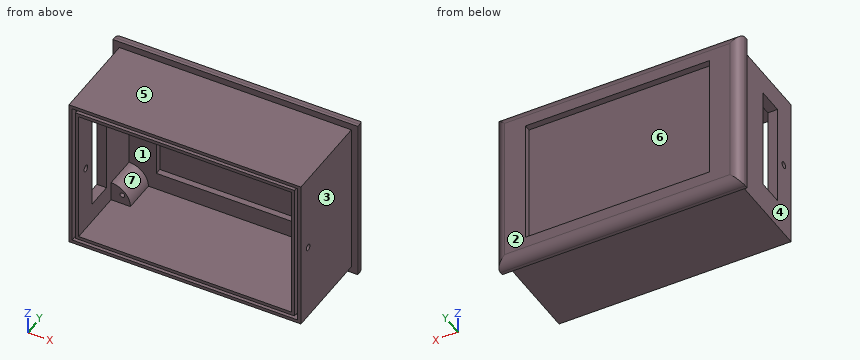
from build123d import *

# Parameters (mm, degrees)
SKETCH1_W                                 = 120.65
SKETCH1_H                                 = 82.55
MAINBODY_DEPTH                            = 50.8
SKETCH2_W                                 = 90.552524
SKETCH2_H                                 = 61.977524
SOLARPANELRECESS_DEPTH                    = 3.175
SKETCH3_W                                 = 77.852524
SKETCH3_H                                 = 49.277524
SOLARPANELWIRINGRECESS_DEPTH              = 88.240311067
SKETCH4_W                                 = 127
SKETCH4_H                                 = 88.9
SKETCH4_W_2                               = 120.65
SKETCH4_H_2                               = 82.55
SKETCH4_W_3                               = 114.3
SKETCH4_H_3                               = 76.2
SKETCH4_W_4                               = 104.775
SKETCH4_H_4                               = 66.675
SKETCH4_W_5                               = 77.852524
SKETCH4_H_5                               = 49.277524
INSIDEENCLOSURERECESS_OUTSIDEFLANGE_DEPTH = 44.45
TOPFANCYFILLET_R                          = 4.7625
CABLEACCESS_REACH                         = 136.479
SKETCH9_R                                 = 1.5875
TOPEDGEHOLES_DEPTH                        = 135.479148012
CORNERSTANDOFFS_DEPTH                     = 15.875
SKETCH11_R                                = 1.143
SCREWSTANDOFFHOLES_DEPTH                  = 6.35
SKETCH12_W                                = 111.125
SKETCH12_H                                = 73.025
SKETCH12_W_2                              = 107.95
SKETCH12_H_2                              = 69.85
WEATHERSEALRECESS_DEPTH                   = 3.175
SKETCH13_W                                = 90.552524
SKETCH13_H                                = 61.977524
BLANKINSERT_BETTERBRIDGING_DEPTH          = 0.125


with BuildPart() as part:
    # Sketch1 → MainBody (new body)
    with BuildSketch(Plane(origin=(0, 0, 0), x_dir=(1, 0, 0), z_dir=(0, 1, 0))):
        Rectangle(SKETCH1_W, SKETCH1_H)
    extrude(amount=MAINBODY_DEPTH)

    # Sketch2 → SolarPanelRecess (cut)
    with BuildSketch(Plane(origin=(0, 50.8, 0), x_dir=(1, 0, 0), z_dir=(0, 1, 0))):
        Rectangle(SKETCH2_W, SKETCH2_H)
    extrude(amount=-SOLARPANELRECESS_DEPTH, mode=Mode.SUBTRACT)

    # Sketch3 → SolarPanelWiringRecess (cut, through all)
    with BuildSketch(Plane(origin=(0, 47.625, 0), x_dir=(1, 0, 0), z_dir=(0, 1, 0))):
        Rectangle(SKETCH3_W, SKETCH3_H)
    extrude(amount=-SOLARPANELWIRINGRECESS_DEPTH, mode=Mode.SUBTRACT)

    # Sketch4 → InsideEnclosureRecess_OutsideFlange (cut)
    with BuildSketch(Plane.XZ):
        Rectangle(SKETCH4_W, SKETCH4_H)
        Rectangle(SKETCH4_W_2, SKETCH4_H_2, mode=Mode.SUBTRACT)
        Rectangle(SKETCH4_W_2, SKETCH4_H_2)
        Rectangle(SKETCH4_W_3, SKETCH4_H_3, mode=Mode.SUBTRACT)
        Rectangle(SKETCH4_W_4, SKETCH4_H_4)
        Rectangle(SKETCH4_W_5, SKETCH4_H_5, mode=Mode.SUBTRACT)
    extrude(amount=-INSIDEENCLOSURERECESS_OUTSIDEFLANGE_DEPTH, mode=Mode.SUBTRACT)

    # TopFancyFillet
    topfancyfillet_edges = [part.edges().sort_by_distance(p)[0] for p in [
        (-60.325, 50.8, 0),
        (0, 50.8, 41.275),
        (60.325, 50.8, 0),
        (0, 50.8, -41.275),
    ]]
    fillet(topfancyfillet_edges, radius=TOPFANCYFILLET_R)

    # Sketch6 → CableAccess (cut, up to next)
    with BuildSketch(Plane.ZY.offset(57.15), mode=Mode.PRIVATE) as cableaccess_sk1:
        Polygon((-14.2875, 24.60625), (14.2875, 24.60625), (26.9875, 24.60625), (26.9875, 11.90625), (-23.8125, 11.90625), (-23.8125, 24.60625), align=None)
    cableaccess_tool1 = extrude(cableaccess_sk1.sketch, amount=-CABLEACCESS_REACH, mode=Mode.PRIVATE) & part.part
    add(cableaccess_tool1.solids().sort_by_distance((-57.15, 18.25625, 1.5875))[0], mode=Mode.SUBTRACT)

    # Sketch9 → TopEdgeHoles (cut, through all)
    with BuildSketch(Plane(origin=(57.15, 0, 0), x_dir=(0, 0, -1), z_dir=(1, 0, 0))):
        with Locations((0, 6.35)):
            Circle(SKETCH9_R)
    extrude(amount=-TOPEDGEHOLES_DEPTH, mode=Mode.SUBTRACT)

    # Sketch10 → CornerStandoffs (add)
    with BuildSketch(Plane.XZ.offset(-44.45)):
        with BuildLine():
            Line((-42.8625, 33.3375), (-52.3875, 33.3375))
            Line((-52.3875, 33.3375), (-52.3875, 23.8125))
            ThreePointArc((-52.3875, 23.8125), (-45.652307909, 26.602307909), (-42.8625, 33.3375))
        make_face()
        with BuildLine():
            ThreePointArc((-42.8625, -33.3375), (-45.652307909, -26.602307909), (-52.3875, -23.8125))
            Line((-52.3875, -23.8125), (-52.3875, -33.3375))
            Line((-52.3875, -33.3375), (-42.8625, -33.3375))
        make_face()
        with BuildLine():
            Line((52.3875, 33.3375), (42.8625, 33.3375))
            ThreePointArc((42.8625, 33.3375), (45.652307909, 26.602307909), (52.3875, 23.8125))
            Line((52.3875, 23.8125), (52.3875, 33.3375))
        make_face()
        with BuildLine():
            ThreePointArc((52.3875, -23.8125), (45.652307909, -26.602307909), (42.8625, -33.3375))
            Line((42.8625, -33.3375), (52.3875, -33.3375))
            Line((52.3875, -33.3375), (52.3875, -23.8125))
        make_face()
    extrude(amount=CORNERSTANDOFFS_DEPTH)

    # Sketch11 → ScrewStandoffHoles (cut)
    with BuildSketch(Plane.XZ.offset(-28.575)):
        with Locations(Location((46.83125, -28.575, 0), (0, 0, 270))):
            Circle(SKETCH11_R)
        with Locations(Location((-46.83125, -28.575, 0), (0, 0, 270))):
            Circle(SKETCH11_R)
        with Locations(Location((-46.83125, 28.575, 0), (0, 0, 270))):
            Circle(SKETCH11_R)
        with Locations(Location((46.83125, 28.575, 0), (0, 0, 270))):
            Circle(SKETCH11_R)
    extrude(amount=-SCREWSTANDOFFHOLES_DEPTH, mode=Mode.SUBTRACT)

    # Sketch12 → WeatherSealRecess (cut)
    with BuildSketch(Plane.XZ):
        Rectangle(SKETCH12_W, SKETCH12_H)
        Rectangle(SKETCH12_W_2, SKETCH12_H_2, mode=Mode.SUBTRACT)
    extrude(amount=-WEATHERSEALRECESS_DEPTH, mode=Mode.SUBTRACT)

    # Sketch13 → BlankInsert_BetterBridging (add)
    with BuildSketch(Plane(origin=(0, 47.625, 0), x_dir=(1, 0, 0), z_dir=(0, 1, 0))):
        Rectangle(SKETCH13_W, SKETCH13_H)
    extrude(amount=-BLANKINSERT_BETTERBRIDGING_DEPTH)


solid = part.part
Design review of the part built by this model. Coordinates are the model's own, in mm. Face numbers are marked on the shaded views. A direction names the side the tool comes from. Round coordinates to 2 decimals unless told otherwise and drop trailing zeros. Write each loop counter-clockwise with the first axis right and the second up, starting at its lowest first coordinate (ties: lowest second). Pieces come first, ordered by that corner, then holes. Notation, with made-up numbers: (56, 88.25) -> (105, 88.25) arc R12 ccw to (105, 107.25) -> close; hole circle Ø7 at (46, -25). An arc over 180 degrees is marked (long way). One line per item, written item: value. Start each with the question number.
Q1. Tool access review of the marked faces 4, 5, 6 and 7: name each direction out of +Z, -Z, +X, -X, +Y, -Y from which nothing blocks a thin tool from reaching the whole face with its end or side.
Q2. To check wall thickness, follow probe 1 along X at (y, z) = (4, -0.5); probe 2 along Z at (x, y) = (-42.5, 6.5); probe 3 along Y at (x, z) = (-9, 36) (3 decimals). State the ranges of each line that lie inside material, in increasing order.
Q3. Insertion check: P1, Ø3.5, axis at y = 1.5, z = -9.5, coming from the +X side; P2, Ø10, axis at x = 28.5, z = 7.5, coming from the -Y side; P3, Ø1.1, axis at x = 47, z = 29, coming from the -Y side (3 decimals); P4, Ø10.5, axis at x = 50, z = -29.5, coming from the -Y side. Each pin has a flat end and moves straight along its axis. Give the tip position at first contact, or say it passes through.
Q4. Add section D-D (y = 6.35). Give the boundary of the cut face in (x, z).
Q5. The part is to be moulded in two halves that separate along X. For the marked faces 1, 2 and 3, say which applies: pulls with the +X half, pulls with the -X half, needs draft (parallel to the pull), parting line crosses it, or undercut.
Response:
1. face 4: +Z, -Z, -X, -Y
1. face 5: +Z, +X, -X, -Y
1. face 6: +Y
1. face 7: -Y
2. probe 1: x = -57.15 to -52.39, 52.39 to 57.15
2. probe 2: z = -38.1 to -33.34, 33.34 to 38.1
2. probe 3: y = 3.175 to 50.8
3. P1: stops at x = 57.15
3. P2: stops at y = 47.5
3. P3: stops at y = 34.925
3. P4: stops at y = 0
4. outline: (-57.15, -38.1) -> (57.15, -38.1) -> (57.15, -1.59) -> (52.39, -1.59) -> (52.39, -33.34) -> (-52.39, -33.34) -> (-52.39, -1.59) -> (-57.15, -1.59) -> close; (-57.15, 1.59) -> (-52.39, 1.59) -> (-52.39, 33.34) -> (52.39, 33.34) -> (52.39, 1.59) -> (57.15, 1.59) -> (57.15, 38.1) -> (-57.15, 38.1) -> close
5. face 1: undercut
5. face 2: needs draft
5. face 3: pulls with the +X half
